Design review of the part built by this model. Coordinates are the model's own, in mm. A direction names the side the tool comes from. Round coordinates to 2 decimals unless told otherwise and drop trailing zeros. Loops run counter-clockwise (first coordinate to the right, second up) from the corner with the lowest first, then second, coordinate; pieces in that order, holes last. Notation, with made-up numbers: M 59.25,48.25 L 82.25,48.25 A11 ccw 82.25,55.25 Z; hole C 4.5,-2 d3. An arc over 180 degrees is marked long. One line per item, written item: value. Start each with the question number.
Item 1: We need section A-A (x = -30). Write out the cut boundary in (y, z), then the cut area to 3 significant figures.
Item 2: We need section C-C (z = 8). State how many separate pieces and enclosed holes the cut face has, then the cut area to 4 significant figures.
Item 3: We need section B-B (y = 9). Write out the cut boundary in (x, z).
Item 4: For faces 4 (the cylindrical face through (-11.112, -9.77, 1.521)), 5 (the flat face through (44.188, 23.658, 7.93)), list the 3-axis set-ups (+Z, -Z, +X, -X, +Y, -Y) from which the entire face can be reached by the end or side of a thin tool; tool diameter is ignored.
Item 5: For line 1 along Y through (x, z) = (-8.5, 8.25); line 2 along X through (y, z) = (4, 7.25); line 3 along X through (y, z) = (29, 8), list the stretches that pass through material, from the lowest coordinate up.
Item 6: Mouldability with a two-part tool opening along X and no side actions: class faces 1 (the cylindrical face through (-35.52, -31.13, 6.59)), 2 (the flat face through (4, 33, 13)), 3 (the cylindrical face through (31.6, 31.2, 8.3)) as released by +X, released by -X, zero draft, split by the parting line, or undercut.
Item 7: We need section D-D (y = 25.5). Write out the cut boundary in (x, z), then the cut area to 3 significant figures.
from build123d import *

# Parameters (mm, degrees)
BOSS_EXTRU_1_DEPTH        = 13
COQUE1_T                  = -5
COQUE1_THICKNESS_2_FACE_W = 90
COQUE1_THICKNESS_2_FACE_H = 65
COQUE1_THICKNESS_2_DEPTH  = 2
ENL_V_MAT_EXTRU_1_REACH   = 110.96
ESQUISSE2_R               = 2.5
ENL_V_MAT_EXTRU_2_REACH   = 95.396
ESQUISSE3_R               = 2.5
ESQUISSE4_W               = 18
ESQUISSE4_H               = 18
ESQUISSE4_W_2             = 15
ESQUISSE4_H_2             = 15
BOSS_EXTRU_2_DEPTH        = 10
ESQUISSE6_R               = 11.5
ESQUISSE6_R_2             = 14.5
ENL_V_MAT_EXTRU_4_DEPTH   = 13
ESQUISSE7_R               = 5
ENL_V_MAT_EXTRU_5_DEPTH   = 3


with BuildPart() as part:
    # Esquisse1 → Boss.-Extru.1 (new body)
    with BuildSketch(Plane.XY):
        Polygon((44.118436308, 33.728448276), (54.118436308, 33.728448276), (54.118436308, 23.728448276), (54.118436308, -41.271551724), (-45.881563692, -41.271551724), (-45.881563692, 33.728448276), align=None)
    extrude(amount=BOSS_EXTRU_1_DEPTH)

    # Coque1
    coque1_openings = [part.faces().sort_by_distance(p)[0] for p in [
        (4.118436308, -3.771551724, 13),
    ]]
    offset(amount=COQUE1_T, openings=coque1_openings, kind=Kind.INTERSECTION)

    # Coque1 thickness 2 face (on inner face of the shell) → Coque1 thickness 2 (cut)
    with BuildSketch(Plane(origin=(4.118436308, -3.771551724, 5), x_dir=(-1, 0, 0), z_dir=(0, 0, -1))):
        Rectangle(COQUE1_THICKNESS_2_FACE_W, COQUE1_THICKNESS_2_FACE_H)
    extrude(amount=COQUE1_THICKNESS_2_DEPTH, mode=Mode.SUBTRACT)

    # Enlèv. mat.-Extru.1: up to this face of the body (flat: up to its plane)
    enl_v_mat_extru_1_end = Plane(part.part.faces().sort_by_distance((54.118436308, -3.771551724, 6.5))[0])
    # Esquisse2 → Enlèv. mat.-Extru.1 (cut, up to the picked face)
    with BuildSketch(Plane.ZY.offset(45.881563692), mode=Mode.PRIVATE) as enl_v_mat_extru_1_sk1:
        with Locations(Location((8, -16.271551724, 0), (0, 0, 270))):
            Circle(ESQUISSE2_R)
    enl_v_mat_extru_1_tool1 = split(extrude(enl_v_mat_extru_1_sk1.sketch, amount=-ENL_V_MAT_EXTRU_1_REACH, mode=Mode.PRIVATE), bisect_by=enl_v_mat_extru_1_end, keep=Keep.BOTH, mode=Mode.PRIVATE)
    # Esquisse2 → Enlèv. mat.-Extru.1 (cut, up to the picked face)
    with BuildSketch(Plane.ZY.offset(45.881563692), mode=Mode.PRIVATE) as enl_v_mat_extru_1_sk2:
        with Locations(Location((8, 8.728448276, 0), (0, 0, 270))):
            Circle(ESQUISSE2_R)
    enl_v_mat_extru_1_tool2 = split(extrude(enl_v_mat_extru_1_sk2.sketch, amount=-ENL_V_MAT_EXTRU_1_REACH, mode=Mode.PRIVATE), bisect_by=enl_v_mat_extru_1_end, keep=Keep.BOTH, mode=Mode.PRIVATE)
    add(enl_v_mat_extru_1_tool1.solids().sort_by(Axis((-45.881564, -16.271552, 8), (1, 0, 0)))[0], mode=Mode.SUBTRACT)
    add(enl_v_mat_extru_1_tool2.solids().sort_by(Axis((-45.881564, 8.728448, 8), (1, 0, 0)))[0], mode=Mode.SUBTRACT)

    # Enlèv. mat.-Extru.2: up to this face of the body (flat: up to its plane)
    enl_v_mat_extru_2_end = Plane(part.part.faces().sort_by_distance((4.118436308, 33.728448276, 6.5))[0])
    # Esquisse3 → Enlèv. mat.-Extru.2 (cut, up to the picked face)
    with BuildSketch(Plane.XZ.offset(41.271551724), mode=Mode.PRIVATE) as enl_v_mat_extru_2_sk1:
        with Locations(Location((-20.881563692, 8, 0), (0, 0, 270))):
            Circle(ESQUISSE3_R)
    enl_v_mat_extru_2_tool1 = split(extrude(enl_v_mat_extru_2_sk1.sketch, amount=-ENL_V_MAT_EXTRU_2_REACH, mode=Mode.PRIVATE), bisect_by=enl_v_mat_extru_2_end, keep=Keep.BOTH, mode=Mode.PRIVATE)
    # Esquisse3 → Enlèv. mat.-Extru.2 (cut, up to the picked face)
    with BuildSketch(Plane.XZ.offset(41.271551724), mode=Mode.PRIVATE) as enl_v_mat_extru_2_sk2:
        with Locations(Location((29.118436308, 8, 0), (0, 0, 270))):
            Circle(ESQUISSE3_R)
    enl_v_mat_extru_2_tool2 = split(extrude(enl_v_mat_extru_2_sk2.sketch, amount=-ENL_V_MAT_EXTRU_2_REACH, mode=Mode.PRIVATE), bisect_by=enl_v_mat_extru_2_end, keep=Keep.BOTH, mode=Mode.PRIVATE)
    add(enl_v_mat_extru_2_tool1.solids().sort_by(Axis((-20.881564, -41.271552, 8), (0, 1, 0)))[0], mode=Mode.SUBTRACT)
    add(enl_v_mat_extru_2_tool2.solids().sort_by(Axis((29.118436, -41.271552, 8), (0, 1, 0)))[0], mode=Mode.SUBTRACT)

    # Esquisse4 → Boss.-Extru.2 (add)
    with BuildSketch(Plane.XY.offset(3)):
        with Locations((-36.881563692, -32.271551724)):
            Rectangle(ESQUISSE4_W, ESQUISSE4_H)
        Polygon((49.118436308, 28.728448276), (49.118436308, 18.728448276), (39.118436308, 28.728448276), align=None)
        Polygon((49.118436308, -36.271551724), (49.118436308, -26.271551724), (39.118436308, -36.271551724), align=None)
        with Locations((-33.381563692, 21.228448276)):
            Rectangle(ESQUISSE4_W_2, ESQUISSE4_H_2)
    extrude(amount=BOSS_EXTRU_2_DEPTH)

    # Esquisse6 → Enlèv. mat.-Extru.4 (cut)
    with BuildSketch(Plane.XY.offset(13)):
        with Locations((-45.881563692, 33.728448276)):
            Circle(ESQUISSE6_R)
        with Locations((-45.881563692, -41.271551724)):
            Circle(ESQUISSE6_R_2)
    extrude(amount=-ENL_V_MAT_EXTRU_4_DEPTH, mode=Mode.SUBTRACT)

    # Esquisse7 → Enlèv. mat.-Extru.5 (cut)
    with BuildSketch(Plane.XY.offset(3)):
        with Locations((-15.881563692, -11.271551724)):
            Circle(ESQUISSE7_R)
    extrude(amount=-ENL_V_MAT_EXTRU_5_DEPTH, mode=Mode.SUBTRACT)


solid = part.part
A:
1. outline: M -41.27,0 L 33.73,0 L 33.73,13 L 13.73,13 L 13.73,3 L -23.27,3 L -23.27,13 L -41.27,13 Z
1. area: 605 mm2
2. separate pieces: 8
2. enclosed holes: 0
2. area: 1,675 mm2
3. outline: M -45.88,0 L 54.12,0 L 54.12,5.51 L 49.12,5.51 L 49.12,3 L -40.88,3 L -40.88,5.51 L -45.88,5.51 Z; M -45.88,10.49 L -40.88,10.49 L -40.88,13 L -45.88,13 Z; M 49.12,10.49 L 54.12,10.49 L 54.12,13 L 49.12,13 Z
4. face 4: +Z, -Z
4. face 5: +Z
5. line 1: -41.27 to -36.27, 28.73 to 33.73
5. line 2: -45.88 to -40.88, 49.12 to 54.12
5. line 3: -35.4 to -23.38, -18.38 to 26.62, 31.62 to 54.12
6. face 1: released by -X
6. face 2: zero draft
6. face 3: undercut
7. outline: M -37.85,0 L 54.12,0 L 54.12,13 L 42.35,13 L 42.35,3 L -25.88,3 L -25.88,13 L -37.85,13 Z
7. area: 513 mm2
